The model under review builds one solid part; all positions refer to its coordinate system, in mm. A direction names the side the tool comes from. Give positions to 0.01 mm unless a question says otherwise; leave off trailing zeros. Order: outer loops, then holes, each group sorted by start corner. A loop starts at its lowest first (then second) coordinate and runs counter-clockwise, first axis right, second up.
Autodesk Inventor part; units mm, degrees
ref_plane "YZ Plane" through (0, 0, 0) normal (1, 0, 0) x (0, 1, 0)
ref_plane "XZ Plane" through (0, 0, 0) normal (0, 1, 0) x (-1, 0, 0)
ref_plane "XY Plane" through (0, 0, 0) normal (0, 0, 1) x (1, 0, 0)
sketch "Sketch1" plane through (0, 0, 0) normal (0, 1, 0) x (-1, 0, 0)
  circle A0 centre (0, 0) radius 17.5
  circle A1 centre (0, 0) radius 1.5
  dimension "d0" = 35
  dimension "d1" = 3
extrude "Extrusion1" add sketch "Sketch1" along normal blind 2
sketch "Sketch2" plane through (0, 2, 0) normal (0, 1, 0) x (1, 0, 0)
  circle A0 centre (0, 0) radius 17.5
  circle A1 centre (0, 0) radius 5
  dimension "d4" = 10
extrude "Extrusion2" add sketch "Sketch2" along normal blind 3.8 contours A1
sketch "Sketch3" plane through (0, 5.8, 0) normal (0, 1, 0) x (1, 0, 0)
  circle A0 centre (0, 0) radius 5
  circle A1 centre (0, 0) radius 3
  dimension "d7" = 6
extrude "Extrusion3" cut sketch "Sketch3" against normal blind 3.8 contours A1
sketch "Sketch4" plane through (0, 0, 0) normal (0, -1, 0) x (1, 0, 0)
  circle A0 centre (0, 0) radius 17.5
  circle A1 centre (12.5, 0) radius 1
  line L0 (0, 0) -> (-6.25, 10.8253)
  line L1 (0, 0) -> (12.5, 0) construction
  line L2 (0, 0) -> (-6.25, -10.8253)
  line L3 (0, 0) -> (12.5, 0) construction
  circle A2 centre (-6.25, 10.8253) radius 1
  circle A3 centre (-6.25, -10.8253) radius 1
  dimension "d11" = 2
  dimension "d12" = 120
  dimension "d13" = 120
  dimension "d14" = 2
  dimension "d15" = 2
extrude "Extrusion4" cut sketch "Sketch4" against normal blind 3.8 contours A1 | A2 | A3
properties part number "servo_paka_dolu"
Item 1: Take a section at A-A (x = 0). Give the boundary of the cut face in (y, z).
Values found:
outline: (0, -17.5) - (2, -17.5) - (2, -5) - (5.8, -5) - (5.8, -3) - (2, -3) - (2, -1.5) - (0, -1.5) - close; (0, 1.5) - (2, 1.5) - (2, 3) - (5.8, 3) - (5.8, 5) - (2, 5) - (2, 17.5) - (0, 17.5) - close
Item 2: For faces 1 (the cylindrical face through (-3, 4, 0)), 2 (the flat face through (-4, 0, 0)), list the 3-axis set-ups (+Z, -Z, +X, -X, +Y, -Y) from which the entire face can be reached by the end or side of a thin tool; tool diameter is ignored.
Values found:
face 1: +Y
face 2: +Z, -Z, +X, -X, -Y
Item 3: Take a section at B-B (z = 0). Give the boundary of the cut face in (x, y).
Values found:
outline: (-17.5, 0) - (-1.5, 0) - (-1.5, 2) - (-3, 2) - (-3, 5.8) - (-5, 5.8) - (-5, 2) - (-17.5, 2) - close; (1.5, 0) - (11.5, 0) - (11.5, 2) - (5, 2) - (5, 5.8) - (3, 5.8) - (3, 2) - (1.5, 2) - close; (13.5, 0) - (17.5, 0) - (17.5, 2) - (13.5, 2) - close
Item 4: Draft analysis for pull direction X (two halves, no side actions). For faces 3 (the cylindrical face through (13.887, 0.986, 10.648)), 4 (the cylindrical face through (-7.044, 0.986, 10.217)), 5 (the flat face through (-4, 2, -4)), state which applies: released by +X, released by -X, zero draft, split by the parting line, or undercut.
Values found:
face 3: split by the parting line
face 4: undercut
face 5: zero draft
Item 5: For line 1 (Z direction, x = -6, y = 1.8); line 2 (Z direction, x = -6.25, y = 0.75); line 3 (Y direction, x = 11, z = 9.5), list the stretches that pass through material, from the lowest coordinate up.
Values found:
line 1: z = -16.44 to -11.79, -9.86 to 9.86, 11.79 to 16.44
line 2: z = -16.35 to -11.83, -9.83 to 9.83, 11.83 to 16.35
line 3: y = 0 to 2
Item 6: Clearance check with flat-ended pins moving along their axes: pin 1 Ø2.5 at (x, z) = (-6.25, -10.83) entering from +Y; pin 2 Ø1.6 at (x, z) = (12.5, 0) entering from +Y; pin 3 Ø1.5 at (x, y) = (10.5, 1.5) entering from -Z. State where each tip first meets the part, or that it passes through.
Values found:
pin 1: stops at y = 2
pin 2: passes through
pin 3: stops at z = -14.53
Item 7: Take a section at D-D (y = 1.6). Give the boundary of the cut face in (x, z), and give its area (3 significant figures).
Values found:
outline: circle Ø35 at (0, 0); hole circle Ø2 at (-6.25, -10.83); hole circle Ø2 at (-6.25, 10.83); hole circle Ø3 at (0, 0); hole circle Ø2 at (12.5, 0)
area: 946 mm2
Item 8: Take a section at C-C (x = -6.5). Give the boundary of the cut face in (y, z).
Values found:
outline: (0, -16.25) - (2, -16.25) - (2, -11.79) - (0, -11.79) - close; (0, -9.86) - (2, -9.86) - (2, 9.86) - (0, 9.86) - close; (0, 11.79) - (2, 11.79) - (2, 16.25) - (0, 16.25) - close
